Source: CAD feature listing. Evaluate the final solid. Frame: model axes, mm. A direction names the side the tool comes from. Give positions to 0.01 mm unless a question says otherwise; leave off trailing zeros. Loops run counter-clockwise (first coordinate to the right, second up) from the corner with the lowest first, then second, coordinate; pieces in that order, holes last.
```python
from build123d import *

# Parameters (mm, degrees)
F0_W     = 80
F0_H     = 80
F0_W_2   = 70
F0_H_2   = 70
F1_DEPTH = 10
F0_W_3   = 60
F0_H_3   = 60
F2_DEPTH = 20
F0_W_4   = 50
F0_H_4   = 50
F3_DEPTH = 30
F0_W_5   = 40
F0_H_5   = 40
F4_DEPTH = 40
F0_W_6   = 30
F0_H_6   = 30
F5_DEPTH = 50
F0_W_7   = 20
F0_H_7   = 20
F6_DEPTH = 60
F0_W_8   = 10
F0_H_8   = 10
F7_DEPTH = 70
F8_DEPTH = 80


with BuildPart() as f1:
    # F0 (on Top) → F1 (new body)
    with BuildSketch(Plane.XY):
        Rectangle(F0_W, F0_H)
        Rectangle(F0_W_2, F0_H_2, mode=Mode.SUBTRACT)
    extrude(amount=F1_DEPTH)

    # F0 (on Top) → F2 (join)
    with BuildSketch(Plane.XY):
        Rectangle(F0_W_2, F0_H_2)
        Rectangle(F0_W_3, F0_H_3, mode=Mode.SUBTRACT)
    extrude(amount=F2_DEPTH)

    # F0 (on Top) → F3 (join)
    with BuildSketch(Plane.XY):
        Rectangle(F0_W_3, F0_H_3)
        Rectangle(F0_W_4, F0_H_4, mode=Mode.SUBTRACT)
    extrude(amount=F3_DEPTH)

    # F0 (on Top) → F4 (join)
    with BuildSketch(Plane.XY):
        Rectangle(F0_W_4, F0_H_4)
        Rectangle(F0_W_5, F0_H_5, mode=Mode.SUBTRACT)
    extrude(amount=F4_DEPTH)

    # F0 (on Top) → F5 (join)
    with BuildSketch(Plane.XY):
        Rectangle(F0_W_5, F0_H_5)
        Rectangle(F0_W_6, F0_H_6, mode=Mode.SUBTRACT)
    extrude(amount=F5_DEPTH)

    # F0 (on Top) → F6 (join)
    with BuildSketch(Plane.XY):
        Rectangle(F0_W_6, F0_H_6)
        Rectangle(F0_W_7, F0_H_7, mode=Mode.SUBTRACT)
    extrude(amount=F6_DEPTH)

    # F0 (on Top) → F7 (join)
    with BuildSketch(Plane.XY):
        Rectangle(F0_W_7, F0_H_7)
        Rectangle(F0_W_8, F0_H_8, mode=Mode.SUBTRACT)
    extrude(amount=F7_DEPTH)

    # F0 (on Top) → F8 (join)
    with BuildSketch(Plane.XY):
        Rectangle(F0_W_8, F0_H_8)
    extrude(amount=F8_DEPTH)


solid = f1.part
```
(1) Ray query, line 1 along Y through (x, z) = (-2, 28); line 2 along X through (y, z) = (-24.5, 14.5); line 3 along Z through (x, y) = (23, 16). Return the intervals inside material, ascending.
A:
line 1: y = -30 to 30
line 2: x = -35 to 35
line 3: z = 0 to 40
(2) Section C-C, the plane z = 44.5. Return the cut outline in (x, y).
A:
outline: (-20, -20) - (20, -20) - (20, 20) - (-20, 20) - close
(3) First-contact query: pin 1 (5 mm diameter, centred on y = 6.5, z = 25.5, fed in from -X); pin 2 (5 mm diameter, centred on y = 1.5, z = 56.5, fed in from -X); pin 3 (3 mm diameter, centred on y = 15, z = 23.5, fed in from +X). Flat tips, straight axial feed; report the tip coordinate or a pass-through.
A:
pin 1: stops at x = -30
pin 2: stops at x = -15
pin 3: stops at x = 30
(4) Section A-A, the plane x = -33. Return the cut outline in (y, z), then the cut area to 3 significant figures.
A:
outline: (-40, 0) - (40, 0) - (40, 10) - (35, 10) - (35, 20) - (-35, 20) - (-35, 10) - (-40, 10) - close
area: 1,500 mm2
(5) Reachability of faces 1 (the flat face through (0, 10, 65)), 2 (the flat face through (0, -30, 25)), 3 (the flat face through (-1, -40, 5)), 4 (the flat face through (-25, 0, 35)), 5 (the flat face through (5, 0, 75)) from +Z, -Z, +X, -X, +Y, -Y: full face, straight path, thin tool, end or side. Return the list, or none.
A:
face 1: +Z, +X, -X, +Y
face 2: +Z, +X, -X, -Y
face 3: +Z, -Z, +X, -X, -Y
face 4: +Z, -X, +Y, -Y
face 5: +Z, +X, +Y, -Y
(6) Section B-B, the plane y = -22. Return the cut outline in (x, z), then the cut area to 3 significant figures.
A:
outline: (-40, 0) - (40, 0) - (40, 10) - (35, 10) - (35, 20) - (30, 20) - (30, 30) - (25, 30) - (25, 40) - (-25, 40) - (-25, 30) - (-30, 30) - (-30, 20) - (-35, 20) - (-35, 10) - (-40, 10) - close
area: 2,600 mm2
